from build123d import *

# Parameters (mm, degrees)
BOSS_EXTRUDE1_DEPTH = 200


with BuildPart() as part:
    # Sketch1 → Boss-Extrude1 (new body)
    with BuildSketch(Plane.XY.offset(116.106580091)):
        Polygon((-39.550290087, 5.294235639), (-36.889629915, 7.954895811), (-36.889629915, 10.362002592), (-31.010950259, 10.362002592), (-31.010950259, 7.954895811), (-28.350290087, 5.294235639), (-28.350290087, 0.029769545), (-31.010950259, -2.630890626), (-31.010950259, -5.037997408), (-36.889629915, -5.037997408), (-36.889629915, -2.630890626), (-39.550290087, 0.029769545), align=None)
    extrude(amount=BOSS_EXTRUDE1_DEPTH)


solid = part.part
Can you work these out from the model? Positions are in its coordinate system, mm. Round coordinates to 2 decimals unless told otherwise and drop trailing zeros. Loops run counter-clockwise (first coordinate to the right, second up) from the corner with the lowest first, then second, coordinate; pieces in that order, holes last. Notation, with made-up numbers: (53, -10.75) - (80, -10.75) arc R6 ccw to (80, -0.75) - close; hole circle Ø3 at (6.5, 79). An arc over 180 degrees is marked (long way). Write item = value, one per line. Start each with the question number.
(1) If I drill on probe 1 along X at (y, z) = (9.5, 268); probe 2 along X at (y, z) = (0, 200); probe 3 along Y at (x, z) = (-37.5, 259), over which ranges is the centre line in solid material (lowest first)? Write a range as [from, to].
(2) If we section it at A-A (z = 143.5): Please give me the cut outline in (x, y), and give its area (3 significant figures).
(3) For P1, Ø0.7, axis at y = -4, z = 259.5, coming from the -X side; P2, Ø2.5, axis at y = 9, z = 264, coming from the -X side; P3, Ø2.5, axis at y = 9.5, z = 256, coming from the +X side, each with a flat end and sliding along its axis, tell me the tip position at first contact or that it passes through.
Ans:
q1.probe_1 = [-36.89, -31.01]
q1.probe_2 = [-39.52, -28.38]
q1.probe_3 = [-2.02, 7.34]
q2.outline = (-39.55, 0.03) - (-36.89, -2.63) - (-36.89, -5.04) - (-31.01, -5.04) - (-31.01, -2.63) - (-28.35, 0.03) - (-28.35, 5.29) - (-31.01, 7.95) - (-31.01, 10.36) - (-36.89, 10.36) - (-36.89, 7.95) - (-39.55, 5.29) - close
q2.area = 133 mm²
q3.P1 = -36.89
q3.P2 = -37.09
q3.P3 = -31.01
